Autodesk Inventor part; units mm, degrees
ref_plane "YZ Plane" through (0, 0, 0) normal (1, 0, 0) x (0, 1, 0)
ref_plane "XZ Plane" through (0, 0, 0) normal (0, 1, 0) x (-1, 0, 0)
ref_plane "XY Plane" through (0, 0, 0) normal (0, 0, 1) x (1, 0, 0)
sketch "Esquisse1" plane through (0, 0, 0) normal (0, 0, 1) x (1, 0, 0)
  line L0 (-6, -3.95) -> (6, -3.95)
  line L1 (6, -3.95) -> (6, 3.95)
  line L2 (6, 3.95) -> (-6, 3.95)
  line L3 (-6, 3.95) -> (-6, -3.95)
  line L4 (-6, -3.95) -> (6, 3.95) construction
  line L5 (6, -3.95) -> (-6, 3.95) construction
  point P0 (0, 0)
  dimension "d0" = 7.9
  dimension "d1" = 12
extrude "Extrusion1" add sketch "Esquisse1" along normal mid plane 600
sketch "Esquisse2" plane through (0, 0, 300) normal (0, 0, 1) x (1, 0, 0)
  line L0 (6, -3.95) -> (6, 3.95)
  line L1 (6, 0.95) -> (4.55, 0.95)
  line L2 (4.3, 1.2) -> (4.3, 1.7)
  line L3 (4.55, 1.95) -> (6, 1.95)
  line L4 (6, 1.95) -> (6, 0.95)
  line L5 (-6, 3.95) -> (-6, -3.95)
  line L6 (-6, 0.95) -> (-4.55, 0.95)
  line L7 (-4.3, 1.2) -> (-4.3, 1.7)
  line L8 (-4.55, 1.95) -> (-6, 1.95)
  line L9 (-6, 1.95) -> (-6, 0.95)
  line L10 (-6, 3.95) -> (6, 3.95)
  arc A0 (-4.55, 0.95) -> (-4.3, 1.2) centre (-4.55, 1.2) ccw
  arc A1 (-4.3, 1.7) -> (-4.55, 1.95) centre (-4.55, 1.7) ccw
  arc A2 (4.3, 1.2) -> (4.55, 0.95) centre (4.55, 1.2) ccw
  arc A3 (4.55, 1.95) -> (4.3, 1.7) centre (4.55, 1.7) ccw
  point P0 (0, 0)
  point P1 (-4.3, 1.95)
  dimension "d4" = 8.6
  dimension "d5" = 4.3
  dimension "d6" = 1
  dimension "d7" = 2
  dimension "d8" = 0.25
extrude "Extrusion2" cut sketch "Esquisse2" against normal through all
fillet "Congé1" radius 0.5 4 edges at (6, 1.95, 0) (6, 0.95, 0) (-6, 0.95, 0) (-6, 1.95, 0)
sketch "Esquisse3" plane through (-6, 3.95, 300) normal (0, 1, 0) x (1, 0, 0)
  line L0 (12, 0) -> (0, 0)
  point P0 (6, 300)
  point P1 (6, 11.6)
  dimension "d12" = 11.6
hole "Perçage1" at (0, 3.95, 288.4) direction (0, -1, 0) diameter 3.5 end through all counterbore diameter 6 counterbore depth 5
pattern_linear "Réseau rectangulaire1" count 24 spacing 25 along (0, 0, -1) of "Perçage1"
properties part number "Rail" material "Acier"
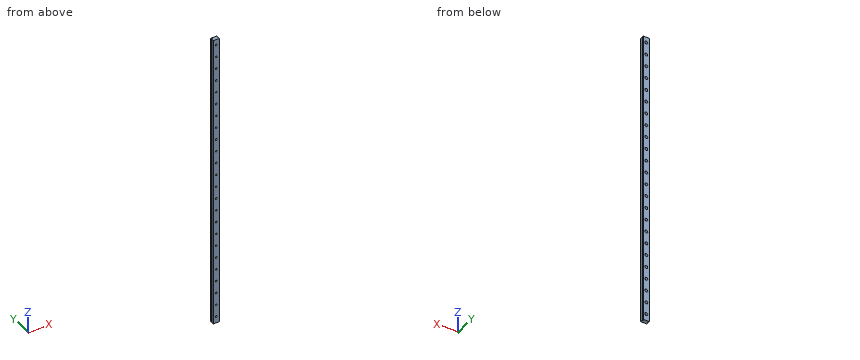
Read the model definition and answer for the solid it produces. Units are mm, in the model's axes. Round coordinates to 2 decimals unless told otherwise and drop trailing zeros. Write each loop counter-clockwise with the first axis right and the second up, starting at its lowest first coordinate (ties: lowest second). Pieces come first, ordered by that corner, then holes. Notation, with made-up numbers: (55.5, -3.5) - (85.5, -3.5) arc R32 ccw to (85.5, 26.5) - close; hole circle Ø9 at (-18, 15). An arc over 180 degrees is marked (long way). One line per item, written item: value.
Q1. Find section B-B (z = 255). Determine the outline of the cut face in (x, y).
The answers:
outline: (-6, -3.95) - (6, -3.95) - (6, 0.45) arc R0.5 ccw to (5.5, 0.95) - (4.55, 0.95) arc R0.25 cw to (4.3, 1.2) - (4.3, 1.7) arc R0.25 cw to (4.55, 1.95) - (5.5, 1.95) arc R0.5 ccw to (6, 2.45) - (6, 3.95) - (-6, 3.95) - (-6, 2.45) arc R0.5 ccw to (-5.5, 1.95) - (-4.55, 1.95) arc R0.25 cw to (-4.3, 1.7) - (-4.3, 1.2) arc R0.25 cw to (-4.55, 0.95) - (-5.5, 0.95) arc R0.5 ccw to (-6, 0.45) - close
Q2. Find section A-A (y = -2.5). Count the separate pieces of the cut face and the enclosed holes in it, and give its area (3 significant figures).
The answers:
separate pieces: 1
enclosed holes: 24
area: 6,970 mm2
Q3. Straight lines are drawn through the part: line 1 (Y direction, x = -4.5, z = -31.5); line 2 (X direction, y = -1.85, z = 13.4); line 3 (Y direction, x = -5.25, z = 162.5). For each, find the intervals that lie inside material, in ascending order. Write a range as from..to.
The answers:
line 1: y = -3.95..0.96, 1.94..3.95
line 2: x = -6..-1.75, 1.75..6
line 3: y = -3.95..0.95, 1.95..3.95
Q4. Each of these flat-tipped pins is pushed along its axis until it touches: P1, Ø3, axis at x = 0.5, z = -12, coming from the +Y side; P2, Ø3, axis at x = 0, z = -286.6, coming from the -Y side. Where does it stop, or does it pass through?
The answers:
P1: stops at y = -1.05
P2: passes through
